Can you work these out from the model? Positions are in its coordinate system, mm. A direction names the side the tool comes from. Give positions to 0.01 mm unless a question says otherwise; leave off trailing zeros. Loops run counter-clockwise (first coordinate to the right, second up) from the corner with the lowest first, then second, coordinate; pieces in that order, holes last. Notation, with made-up numbers: (60.25, 75.5) - (119.25, 75.5) arc R21 cw to (119.25, 98.5) - close; hole circle Ø2 at (68, 83). An arc over 180 degrees is marked (long way). Answer as a JSON object with one key per item and string values.
```python
from build123d import *

# Parameters (mm, degrees)
SKETCH2_R          = 2
CUT_EXTRUDE1_DEPTH = 10
SKETCH3_W          = 25.1
SKETCH3_H          = 3
CHAMFER1_SIZE      = 5
SKETCH4_R          = 1.5
SKETCH4_R_2        = 1.55
SKETCH4_R_3        = 5.5
CUT_EXTRUDE2_DEPTH = 10


with BuildPart() as part:
    # Sketch1 → Revolve1 (revolve)
    with BuildSketch(Plane(origin=(0, 0, 0), x_dir=(1, 0, 0), z_dir=(0, 1, 0))):
        Polygon((15.25, 26.5), (15.25, 23.5), (25.1, 23.5), (25.1, -23.5), (27.1, -23.5), (27.1, 26.5), align=None)
    revolve(axis=Axis((0, 0, -51.288157895), (0, 0, 1)))

    # Sketch2 → Cut-Extrude1 (cut)
    with BuildSketch(Plane(origin=(0, 0, -26.5), x_dir=(-1, 0, 0), z_dir=(0, 0, -1))):
        with Locations((0, 20.25)):
            Circle(SKETCH2_R)
        with Locations((17.537014427, -10.125)):
            Circle(SKETCH2_R)
        with Locations((-17.537014427, -10.125)):
            Circle(SKETCH2_R)
    extrude(amount=-CUT_EXTRUDE1_DEPTH, mode=Mode.SUBTRACT)

    # Sketch3 → Revolve2 (revolve)
    with BuildSketch(Plane(origin=(0, 0, 0), x_dir=(1, 0, 0), z_dir=(0, 1, 0))):
        with Locations((12.55, 8.8)):
            Rectangle(SKETCH3_W, SKETCH3_H)
    revolve(axis=Axis((0, 0, -51.288157895), (0, 0, 1)))

    # Chamfer1
    chamfer1_edges = [part.edges().sort_by_distance(p)[0] for p in [
        (-25.1, 0, -7.3),
        (-25.1, 0, -10.3),
    ]]
    chamfer(chamfer1_edges, length=CHAMFER1_SIZE)

    # Sketch4 → Cut-Extrude2 (cut)
    with BuildSketch(Plane(origin=(0, 0, -10.3), x_dir=(-1, 0, 0), z_dir=(0, 0, -1))):
        with Locations((0, 12.5)):
            Circle(SKETCH4_R)
        with Locations((0, -12.5)):
            Circle(SKETCH4_R)
        with Locations((-8.5, 0)):
            Circle(SKETCH4_R_2)
        with Locations((8.5, 0)):
            Circle(SKETCH4_R_2)
        Circle(SKETCH4_R_3)
    extrude(amount=-CUT_EXTRUDE2_DEPTH, mode=Mode.SUBTRACT)


solid = part.part
```
1) Which directions (+Z, -Z, +X, -X, +Y, -Y) give clear straight access to the entire face, cutting with the end or side of a thin tool? Please do faces 1 (the flat face through (-8, -24, 23.5)), 2 (the cylindrical face through (23.186, -9.613, -19.343)), 3 (the cylindrical face through (-12.1, -9.28, -24.98)), 4 (the cylindrical face through (23.186, -9.613, 10.781)), 5 (the cylindrical face through (-9.978, 0.466, -8.821)).
Check sheet entries:
{"face 1": "+Z, +X, -X, +Y, -Y", "face 2": "none", "face 3": "-Z", "face 4": "+Z", "face 5": "+Z, -Z"}
2) Imagine slicing it at B-B on z = -5. Write out the boundary of the cut face in (x, y).
Check sheet entries:
{"outline": "circle Ø54.2 at (0, 0); hole circle Ø44.8 at (0, 0)"}
3) Imagine slicing it at C-C on z = 9. Write out the boundary of the cut face in (x, y).
Check sheet entries:
{"outline": "circle Ø54.2 at (0, 0); hole circle Ø50.2 at (0, 0)"}
4) If we mould it in two halves opening along X, with no side actions, what happens to faces 6 (the cylindrical face through (25.034, -10.379, -1.85)), 7 (the flat face through (-4, -4, -10.3)), 8 (the flat face through (12, -12, -26.5))? For each: released by +X, released by -X, zero draft, split by the parting line, or undercut.
Check sheet entries:
{"face 6": "split by the parting line", "face 7": "undercut", "face 8": "zero draft"}
5) I need wall thicknesses on L1, parallel to Z at x = -17.5, y = -2; L2, parallel to Y at x = 0, z = 14.25; L3, parallel to X at y = -23, z = -17. Which ranges of each line are inside material? Lowest first, please.
Check sheet entries:
{"L1": "-26.5 to -23.5, -10.3 to -7.3", "L2": "-27.1 to -25.1, 25.1 to 27.1", "L3": "-14.33 to -10.05, 10.05 to 14.33"}
6) Imagine slicing it at A-A on y = 0. Give the number of separate pieces and of enclosed holes in the cut face, and give its area (3 significant figures).
Check sheet entries:
{"separate pieces": "4", "enclosed holes": "0", "area": "408 mm2"}
7) I'm going to push flat-ended pins straight in: P1, Ø12, axis at y = 18, z = -12, coming from the -X side; P2, Ø4.5, axis at x = -17.54, y = -10.12, coming from the -Z side; P3, Ø12, axis at y = -12, z = -12, coming from the -X side; P4, Ø2.5, axis at x = 0, y = 20.25, coming from the +Z side. Where does each tip first touch, or does it pass through?
Check sheet entries:
{"P1": "x = -24.3", "P2": "z = -26.5", "P3": "x = -26.43", "P4": "z = -5.9"}
